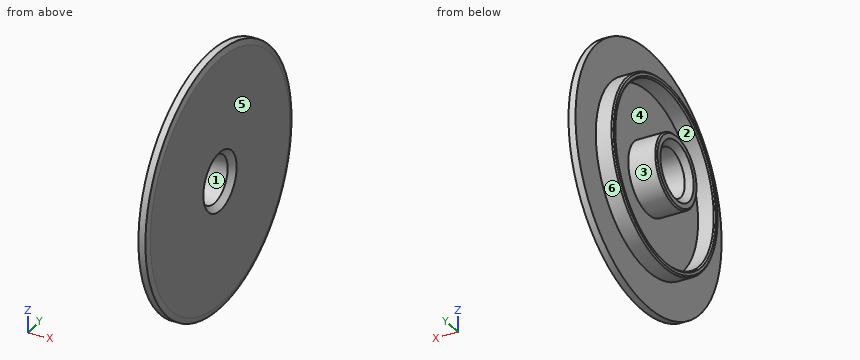
```python
from build123d import *

# Parameters (mm, degrees)
CHAMFER_1_SIZE = 2
CHAMFER_3_SIZE = 0.5


with BuildPart() as part:
    # Эскиз1 → Повернуть1 (revolve)
    with BuildSketch(Plane.XY):
        Polygon((0, 8.25), (13, 8.25), (13, 43), (12.464101615, 45), (10, 45), (10, 32.5), (4, 32.5), (4, 30.5), (10, 30.5), (10, 12.5), (0, 12.5), align=None)
    revolve(axis=Axis((0, 0, 0), (1, 0, 0)))

    # Фаска1
    chamfer_1_edges = [part.edges().sort_by_distance(p)[0] for p in [
        (13, -8.25, 0),
        (0, -8.25, 0),
    ]]
    chamfer(chamfer_1_edges, length=CHAMFER_1_SIZE)

    # Фаска3
    chamfer_3_edges = [part.edges().sort_by_distance(p)[0] for p in [
        (4, -30.5, 0),
        (4, -32.5, 0),
        (0, -12.5, 0),
    ]]
    chamfer(chamfer_3_edges, length=CHAMFER_3_SIZE)


solid = part.part
```
CAD build for the part. Positions are in the model's coordinates, mm. Face numbers are marked on the shaded views. A direction names the side the tool comes from. Coordinates: 2 decimals unless noted, no trailing zeros. Write each loop counter-clockwise with the first axis right and the second up, starting at its lowest first coordinate (ties: lowest second). Pieces come first, ordered by that corner, then holes.
(1) 3-axis set-ups, long thin cutter, end or side, ignore diameter. For the marked faces 1 and 2: which of +Z, -Z, +X, -X, +Y, -Y reach the whole face in a straight line?
(2) Drill centre lines: probe 1 along Z at (x, y) = (7.3, 0); probe 2 along Y at (x, z) = (9, 3.5); probe 3 along Y at (x, z) = (4.5, -10.5). Where is each one in solid material? Low to high.
(3) Cut at C-C, the plane x = 6.5. List the corners of the cut face in (y, z), and give its area (3 significant figures).
(4) Flat gauge pins, fed straight in: pin 1 (4 mm diameter, centred on y = 5.5, z = -0.5, fed in from +X); pin 2 (1 mm diameter, centred on y = -17.5, z = -6, fed in from -X); pin 3 (4 mm diameter, centred on x = 6, y = 10.5, fed in from -Z); pin 4 (2 mm diameter, centred on x = 3.5, z = -12, fed in from +Y). Where does each tip first touch, or does it go through?
(5) Two-plate mould, pull along Y, no slides. Class the marked faces 3, 4, 5 and 6: +Y half, -Y half, draft (parallel to the pull), parting line (faces both ways), or undercut.
Geometry says:
1. face 1: +X, -X
1. face 2: -X
2. probe 1: z = -32.5 to -30.5, -12.5 to -8.25, 8.25 to 12.5, 30.5 to 32.5
2. probe 2: y = -32.31 to -30.3, -12 to -7.47, 7.47 to 12, 30.3 to 32.31
2. probe 3: y = -30.76 to -28.64, -6.78 to 6.78, 28.64 to 30.76
3. outline: circle Ø65 at (0, 0); circle Ø25 at (0, 0); hole circle Ø61 at (0, 0); hole circle Ø16.5 at (0, 0)
3. area: 673 mm2
4. pin 1: passes through
4. pin 2: stops at x = 10
4. pin 3: stops at z = -31.37
4. pin 4: stops at y = 30.27
5. face 3: undercut
5. face 4: undercut
5. face 5: draft
5. face 6: parting line
